Solid Edge part; units mm, degrees
sketch "Sketch1" plane through (0, 0, 0) normal (0, 0, 1) x (1, 0, 0)
  line L0 (6.35, 0) -> (6.35, 76.2)
  line L1 (6.35, 76.2) -> (22.225, 76.2)
  line L2 (22.225, 53.975) -> (22.225, 76.2)
  line L3 (22.225, 53.975) -> (98.425, 53.975)
  line L4 (98.425, 76.2) -> (98.425, 53.975)
  line L5 (98.425, 76.2) -> (114.3, 76.2)
  line L6 (114.3, 76.2) -> (114.3, 0)
  line L7 (114.3, 0) -> (98.425, 0)
  line L8 (98.425, 22.225) -> (98.425, 0)
  line L9 (98.425, 22.225) -> (22.225, 22.225)
  line L10 (22.225, 0) -> (22.225, 22.225)
  line L11 (22.225, 0) -> (6.35, 0)
  dimension "D1" = 6.35
  dimension "D2" = 22.225
  dimension "D3" = 6.35
extrude "Protrusion1" add sketch "Sketch1" along normal blind 12.7
hole "Hole_1" at (14.2875, 0, 6.35) direction (0, 1, 0) diameter 6.35 end through all
hole "Hole1" at (106.3625, 0, 6.35) direction (0, 1, 0) diameter 6.35 end through all
sketch "Sketch2" plane through (63.5, 38.1, 12.7) normal (0, 0, 1) x (1, 0, 0)
  line L0 (28.575, -9.525) -> (-34.925, -9.525)
  line L1 (-34.925, 9.525) -> (28.575, 9.525)
  arc A0 (-34.925, -9.525) -> (-34.925, 9.525) centre (-34.925, 0) cw
  arc A1 (28.575, 9.525) -> (28.575, -9.525) centre (28.575, 0) cw
extrude "Cutout1" cut sketch "Sketch2" against normal through all
fillet "Round_1" radius 12.7 4 edges at (22.225, 22.225, 6.35) (22.225, 53.975, 6.35) (98.425, 53.975, 6.35) (98.425, 22.225, 6.35)
sketch "Sketch3" plane through (60.325, 38.1, 12.7) normal (0, 0, 1) x (1, 0, 0)
  line L0 (-63.5, 38.1) -> (-63.5, -38.1)
  line L1 (-63.5, -38.1) -> (-50.8, -38.1)
  line L2 (-50.8, -38.1) -> (-50.8, 38.1)
  line L3 (-50.8, 38.1) -> (-63.5, 38.1)
  dimension "D1" = 63.5
extrude "ExtrudedProtrusion_2" add sketch "Sketch3" against normal blind 12.7
fillet "Round_2" radius 3.175 8 edges at (22.225, 0, 6.35) (22.225, 76.2, 6.35) (98.425, 76.2, 6.35) (114.3, 76.2, 6.35) (114.3, 0, 6.35) (98.425, 0, 6.35) (-3.175, 76.2, 6.35) (-3.175, 0, 6.35)
hole "Hole_5" at (-3.175, 15.875, 3.81) direction (1, 0, 0) diameter 4.826 depth 7.62
hole "Hole2" at (-3.175, 60.325, 3.81) direction (1, 0, 0) diameter 4.826 depth 7.62
extrude "ExtrudedCutout_2" [suppressed]
fillet "Round_4" [suppressed]
hole "Hole_9" [suppressed]
properties part number "SR-03" material "Polyethylene, low density"
The listing builds one solid part. Answer for the finished solid, in the listing's coordinates (mm). A direction names the side the tool comes from. Give positions to 0.01 mm unless a question says otherwise; leave off trailing zeros. Write each loop counter-clockwise with the first axis right and the second up, starting at its lowest first coordinate (ties: lowest second). Pieces come first, ordered by that corner, then holes. Notation, with made-up numbers: (76.25, -40) - (88.25, -40) arc R17 ccw to (88.25, -16) - close; hole circle Ø4 at (-17, 68). An arc over 180 degrees is marked (long way). One line per question, with ' | ' between items. Start each with the question number.
1. For faces 1 (the face through (99.33, 0.955, 6.439)), 2 (the face through (99.38, 75.295, 6.439)), 3 (the face through (101.598, 37.891, 6.439)), determine the directions among +Z, -Z, +X, -X, +Y, -Y from which every point of the face is accessible in a straight line to the end or side of a thin tool.
2. Determine the mould class of faces 4 (the face through (113.39, 75.25, 6.44)), 5 (the face through (0.69, 62.68, 3.29)), 6 (the face through (-2.27, 75.245, 6.261)), 7 (the face through (22.225, 70, 6)) for opening direction X: +X half, -X half, draft (parallel to the pull), parting line (faces both ways), or undercut.
3. Section D-D, the plane x = 88.5 is taken. Determine the outline of the cut face in (y, z) (3 decimals), then the cut area to 3 significant figures.
4. Given P1, Ø6.5, axis at x = 49.5, z = 6, coming from the +Y side (3 decimals); P2, Ø1, axis at x = 32.5, z = 7, coming from the +Y side; P3, Ø4, axis at x = 69, z = 6.5, coming from the -Y side (3 decimals); P4, Ø4, axis at y = 61, z = 4.5, coming from the -X side (3 decimals), each flat-ended and moving along its own axis, determine where each tip first touches the part or whether it passes through.
5. Section B-B, the plane y = 6 is taken. Count the separate pieces of the cut face and the enclosed holes in it, then the cut area to 3 significant figures.
6. Section A-A, the plane x = 43 is taken. Determine the outline of the cut face in (y, z) (3 decimals).
7. Straight lines are drawn through the part: line 1 (Y direction, x = 2.75, z = 3.81); line 2 (X direction, y = 25, z = 6.35) (1 decimal); line 3 (Y direction, x = 75, z = 2.5) (3 decimals). For each, find the intervals that lie inside material, in ascending order.
Result:
1) face 1: +Z, -Z, -Y | face 2: +Z, -Z, +Y | face 3: +Z, -Z
2) face 4: +X half | face 5: draft | face 6: -X half | face 7: undercut
3) outline: (21.918, 0) - (28.575, 0) - (28.575, 12.7) - (21.918, 12.7) - close; (47.625, 0) - (54.282, 0) - (54.282, 12.7) - (47.625, 12.7) - close | area: 169 mm2
4) P1: stops at y = 53.975 | P2: stops at y = 54.32 | P3: stops at y = 22.225 | P4: stops at x = -3.175
5) separate pieces: 2 | enclosed holes: 2 | area: 461 mm2
6) outline: (22.225, 0) - (28.575, 0) - (28.575, 12.7) - (22.225, 12.7) - close; (47.625, 0) - (53.975, 0) - (53.975, 12.7) - (47.625, 12.7) - close
7) line 1: y = 0 to 13.46, 18.29 to 57.91, 62.74 to 76.2 | line 2: x = -3.2 to 11.1, 17.5 to 103.2, 109.5 to 114.3 | line 3: y = 22.225 to 28.575, 47.625 to 53.975
